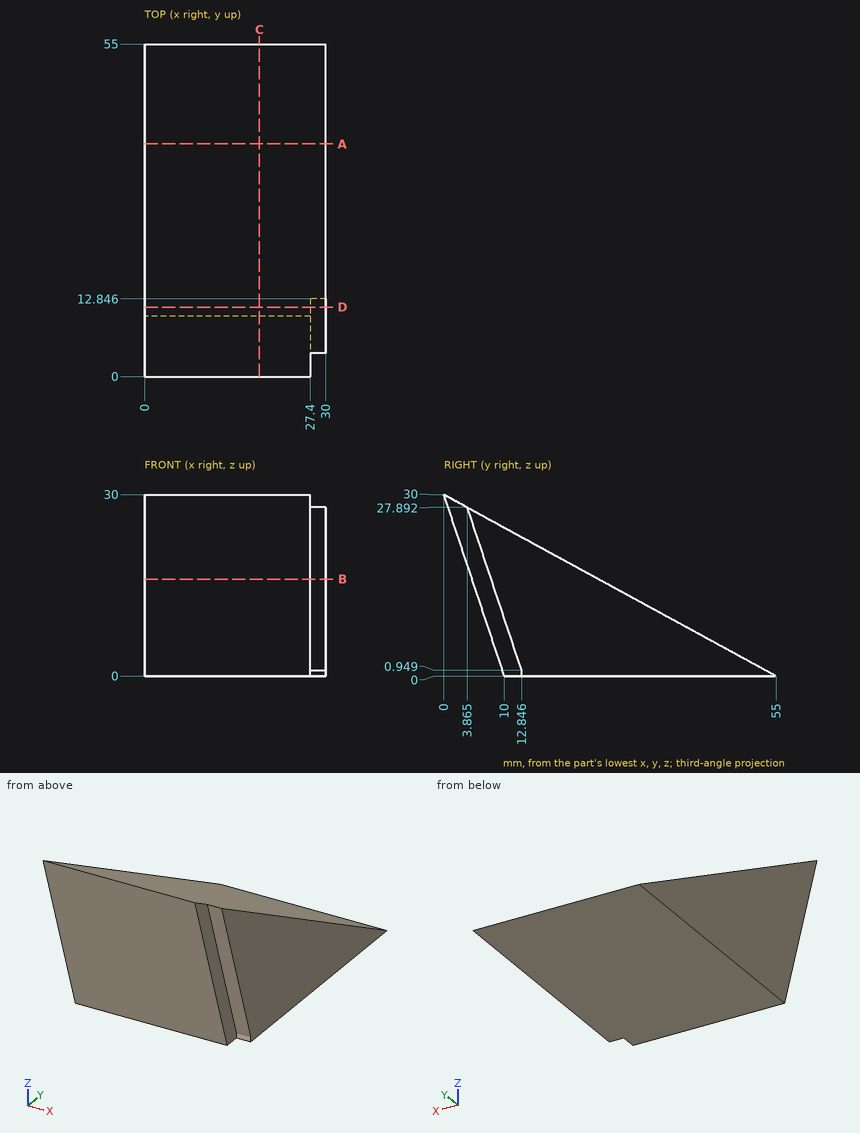
Can you work these out from the drawing? Everything is in mm from the part's minimum corner. Round coordinates to 2 decimals unless told otherwise and drop trailing zeros. Write each loop counter-clockwise with the first axis right and the second up, starting at its lowest first coordinate (ties: lowest second). Pieces come first, ordered by that corner, then holes. Notation, with made-up numbers: (47.5, 6) - (58.5, 6) arc R23 cw to (58.5, 32) - close; hole circle Ø4 at (25.5, 88.5). An arc over 180 degrees is marked (long way). Put each result on its own line as item: value. Start each with the question number.
(1) I want a section at A-A, the plane y = 38.5. Please give me the cut outline in (x, z), plus the area to 3 significant figures.
(2) I want a section at C-C, the plane x = 19. Please give me the cut outline in (y, z).
(3) Will these pins go through, and if not, where does the flat tip stop? pin 1 (1 mm diameter, centred on x = 25.5, z = 22, fed in from +Y) (1 decimal); pin 2 (5 mm diameter, centred on y = 6, z = 6.5, fed in from +X); pin 3 (8 mm diameter, centred on x = 9, y = 42, fed in from +Z).
(4) I need wall thicknesses on probe 1 along Z at (x, y) = (23, 46.5); probe 2 along Z at (x, y) = (25.5, 22.5); probe 3 along Y at (x, z) = (21.5, 10.5). Which ranges of each line are inside material? Lowest first, please.
(5) I want a section at D-D, the plane y = 11.5. Please give me the cut outline in (x, z), plus the area to 3 significant figures.
(6) I want a section at B-B, the plane z = 16. Please give me the cut outline in (x, y), plus the area to 3 significant figures.
Here are the results:
1. outline: (0, 0) - (30, 0) - (30, 9) - (0, 9) - close
1. area: 270 mm^2
2. outline: (0, 30) - (10, 0) - (55, 0) - close
3. pin 1: stops at y = 15.6
3. pin 2: stops at x = 27.4
3. pin 3: stops at z = 9.27
4. probe 1: z = 0 to 4.64
4. probe 2: z = 0 to 17.73
4. probe 3: y = 6.5 to 35.75
5. outline: (0, 0) - (27.4, 0) - (27.4, 4.99) - (30, 4.99) - (30, 23.73) - (0, 23.73) - close
5. area: 699 mm^2
6. outline: (0, 4.67) - (27.4, 4.67) - (27.4, 7.83) - (30, 7.83) - (30, 25.67) - (0, 25.67) - close
6. area: 622 mm^2
